Model file for the job. Use its own axes, mm. Face numbers are marked on the shaded views. A direction names the side the tool comes from. Round coordinates to 2 decimals unless told otherwise and drop trailing zeros. Order: outer loops, then holes, each group sorted by start corner. A loop starts at its lowest first (then second) coordinate and runs counter-clockwise, first axis right, second up. Notation, with made-up numbers: (19.5, 76) -> (37.5, 76) arc R14 ccw to (37.5, 80) -> close; hole circle Ø11 at (20.25, 31). An arc over 180 degrees is marked (long way). Answer as CSV lines item,"result".
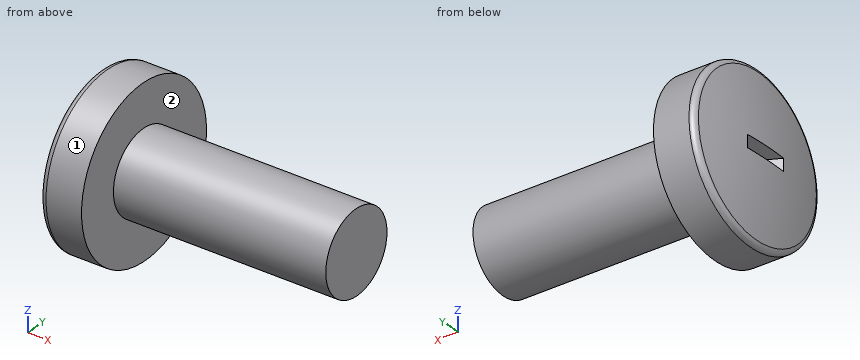
```python
from build123d import *

# Parameters (mm, degrees)
SKETCH3_W = 0.74
SKETCH3_H = 2.9
SKETCH4_W = 0.37
SKETCH4_H = 0.37


with BuildPart() as part:
    # BodySke → Base-Revolve (revolve)
    with BuildSketch(Plane.XY):
        with BuildLine():
            Line((3, 2.4), (3, 4.9))
            Line((3, 4.9), (0.891938874, 4.9))
            ThreePointArc((0.891938874, 4.9), (0.668733198, 4.822452166), (0.541689281, 4.623217923))
            ThreePointArc((0.541689281, 4.623217923), (0.135883931, 2.327421923), (0, 0))
            Line((0, 0), (15.6, 0))
            Line((15.6, 0), (15.6, 2.4))
            Line((15.6, 2.4), (3, 2.4))
        make_face()
    revolve(axis=Axis((-25.4, 0, 0), (1, 0, 0)))

    # Sketch3 → Cut-Loft1 section 0
    with BuildSketch(Plane(origin=(0, 0, 0), x_dir=(0, 0, -1), z_dir=(1, 0, 0))):
        Rectangle(SKETCH3_W, SKETCH3_H)
    # Sketch4 → Cut-Loft1 section 1
    with BuildSketch(Plane(origin=(1.76, 0, 0), x_dir=(0, 0, -1), z_dir=(1, 0, 0))):
        Rectangle(SKETCH4_W, SKETCH4_H)
    loft(mode=Mode.SUBTRACT)


solid = part.part
```
Q1. Saw through at B-B (x = 2.25). Write the cut outline in (y, z), plus the area to 3 significant figures.
Checks:
outline,"circle Ø9.8 at (0, 0)"
area,"75.4 mm²"
Q2. Flat gauge pins, fed straight in: pin 1 (5 mm diameter, centred on y = -2.5, z = 3, fed in from -X); pin 2 (2 mm diameter, centred on x = 9, z = -3.5, fed in from -Y); pin 3 (1 mm diameter, centred on y = 1.5, z = -3.5, fed in from +X); pin 4 (3 mm diameter, centred on x = 8.5, z = -0.5, fed in from +Y). Where does each tip first touch, or does it go through?
Checks:
pin 1,"x = 0.05"
pin 2,"through"
pin 3,"x = 3"
pin 4,"y = 2.4"
Q3. Tool access for the marked faces 1 and 2: list every direction of +Z, -Z, +X, -X, +Y, -Y with a clear straight run to the whole face (end or side of a thin tool).
Checks:
face 1,"+X, -X"
face 2,"+X"
Q4. Saw through at A-A (x = 14). Write the cut outline in (y, z).
Checks:
outline,"circle Ø4.8 at (0, 0)"
Q5. Wall check: L1, parallel to X at y = -1.25, z = 0.75; L2, parallel to X at y = 0.5, z = -4; L3, parallel to Y at x = 7.75, z = -1.25. Give the ranges that are in metal, low to high. Write a range as [from, to].
Checks:
L1,"[0.05, 15.6]"
L2,"[0.41, 3]"
L3,"[-2.05, 2.05]"
